Could you check a few things on this drawing? It's one solid part, dimensions in mm from its lowest x, y, z. A direction names the side the tool comes from. Give positions to 0.01 mm unless a question says otherwise; leave off trailing zeros. Loops run counter-clockwise (first coordinate to the right, second up) from the corner with the lowest first, then second, coordinate; pieces in that order, holes last. Notation, with made-up numbers: (7.25, -16) -> (35.25, -16) arc R30 cw to (35.25, 10) -> close; hole circle Ø1 at (86.25, 9). An arc over 180 degrees is marked (long way). Use CSV: the item, a comma, the result in double quotes.
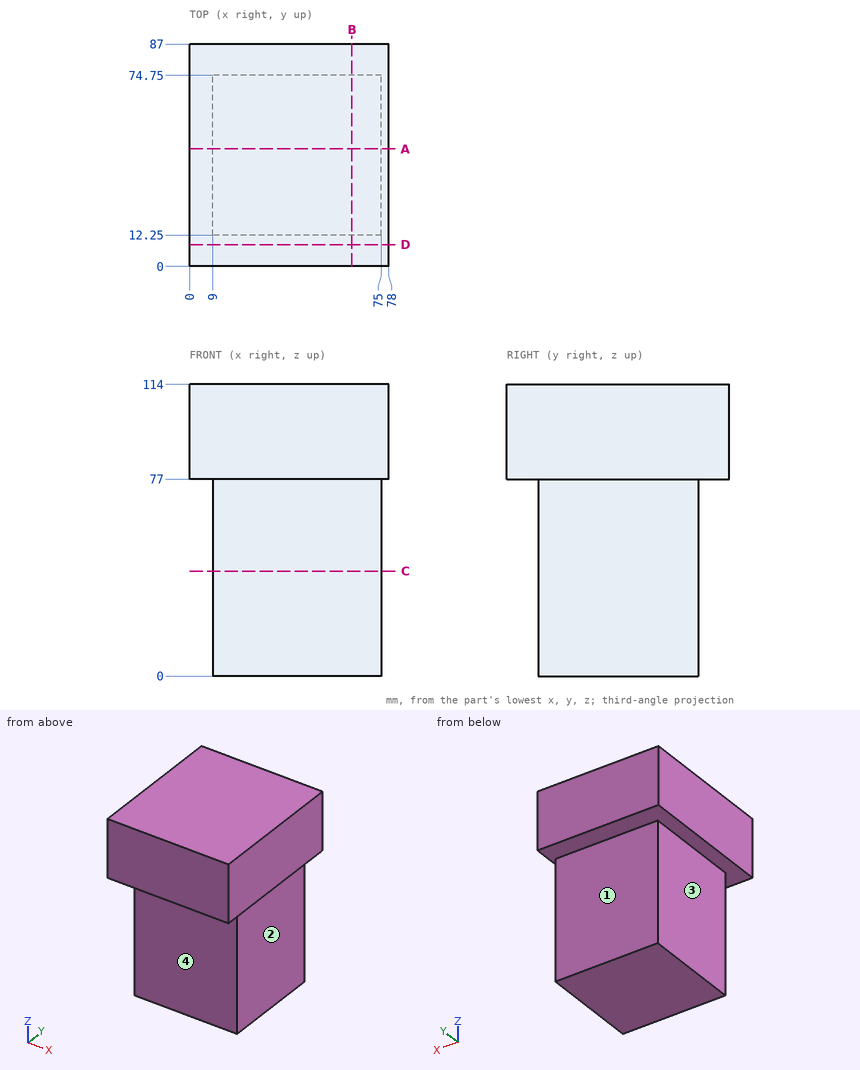
(1) Will these pins go through, and if not, where does the flat tip stop? pin 1 Ø2 at (x, z) = (55, 11.5) entering from -Y; pin 2 Ø3 at (y, z) = (53, 26.5) entering from +X; pin 3 Ø1.5 at (x, z) = (50, 24.5) entering from +Y.
Answer sheet:
pin 1,"stops at y = 12.25"
pin 2,"stops at x = 75"
pin 3,"stops at y = 74.75"
(2) If I drill on L1, parallel to X at y = 36, z = 22.5; L2, parallel to Y at x = 68, z = 57, over which ranges is the centre line in solid material (lowest first)? Write a range as from..to.
Answer sheet:
L1,"x = 9..75"
L2,"y = 12.25..74.75"
(3) Which directions (+Z, -Z, +X, -X, +Y, -Y) give clear straight access to the entire face, cutting with the end or side of a thin tool? Please do the marked faces 1, 2, 3 and 4.
Answer sheet:
face 1,"-Z, +X, -X, +Y"
face 2,"-Z, +X, +Y, -Y"
face 3,"-Z, -X, +Y, -Y"
face 4,"-Z, +X, -X, -Y"
(4) If we section it at B-B, the plane x = 63.5: Write out the boundary of the cut face in (y, z).
Answer sheet:
outline,"(0, 77) -> (12.25, 77) -> (12.25, 0) -> (74.75, 0) -> (74.75, 77) -> (87, 77) -> (87, 114) -> (0, 114) -> close"
(5) If we section it at D-D, the plane y = 8.5: Write out the boundary of the cut face in (x, z), then the cut area to 3 significant figures.
Answer sheet:
outline,"(0, 77) -> (78, 77) -> (78, 114) -> (0, 114) -> close"
area,"2,890 mm2"
(6) If we section it at C-C, the plane z = 41: Write out the boundary of the cut face in (x, y), then the cut area to 4 significant figures.
Answer sheet:
outline,"(9, 12.25) -> (75, 12.25) -> (75, 74.75) -> (9, 74.75) -> close"
area,"4,125 mm2"
(7) If we section it at A-A, the plane y = 46: Write out the boundary of the cut face in (x, z), then the cut area to 3 significant figures.
Answer sheet:
outline,"(0, 77) -> (9, 77) -> (9, 0) -> (75, 0) -> (75, 77) -> (78, 77) -> (78, 114) -> (0, 114) -> close"
area,"7,970 mm2"
